```python
from build123d import *

# Parameters (mm, degrees)
F3_DEPTH = 15
F5_R     = 1
F6_DEPTH = 25


with BuildPart() as f1:
    # F0 (on Front) → F1 (revolve)
    with BuildSketch(Plane.XZ):
        with BuildLine():
            Line((2.6, 15), (2.6, 0))
            Line((2.6, 0), (21.5, 0))
            Line((21.5, 0), (21.5, 1))
            Line((21.5, 1), (20.5, 1))
            ThreePointArc((20.5, 1), (20.146447, 1.146447), (20, 1.5))
            Line((20, 1.5), (20, 13.5))
            ThreePointArc((20, 13.5), (20.146447, 13.853553), (20.5, 14))
            Line((20.5, 14), (21.5, 14))
            Line((21.5, 14), (21.5, 15))
            Line((21.5, 15), (2.6, 15))
        make_face()
    revolve(axis=Axis((0, 0, 3.375067), (0, 0, 1)))

    # F2 (on Top) → F3 (join, through all)
    with BuildSketch(Plane.XY):
        with BuildLine():
            Line((1.661325, -2), (-1.661325, -2))
            ThreePointArc((-1.661325, -2), (0, -2.6), (1.661325, -2))
        make_face()
    extrude(amount=F3_DEPTH)

    # F5 (on face) → F6 (cut)
    with BuildSketch(Plane(origin=(0, 6.5, 6.5), x_dir=(-1, 0, 0), z_dir=(0, 0.707107, 0.707107))):
        with Locations((0, 23.020815)):
            Circle(F5_R)
    extrude(amount=-F6_DEPTH, mode=Mode.SUBTRACT)


solid = f1.part
```
Could you check a few things on this model? Use its own coordinates, in mm. A direction names the side the tool comes from. Coordinates: 2 decimals unless noted, no trailing zeros. Write each loop counter-clockwise with the first axis right and the second up, starting at its lowest first coordinate (ties: lowest second). Pieces come first, ordered by that corner, then holes. Notation, with made-up numbers: (-14, 34) -> (31, 34) arc R28 cw to (31, 72) -> close; hole circle Ø11 at (32.25, 52.5). An arc over 180 degrees is marked (long way). Write item = value, one per line. Start each with the question number.
(1) I want a section at C-C (z = 7.5). Please give me the cut outline in (x, y), plus the area to 3 significant figures.
(2) Will these pins go through, and if not, where does the flat tip stop? pin 1 (1 mm diameter, centred on x = 7.5, z = 11.5, fed in from +Y) (3 decimals); pin 2 (2 mm diameter, centred on y = 8.5, z = 7, fed in from -X); pin 3 (8 mm diameter, centred on x = 2.5, z = 8.5, fed in from +Y).
(3) I need wall thicknesses on line 1 (Y direction, x = 0, z = 4); line 2 (X direction, y = 0, z = 11.25); line 3 (Z direction, x = -19, y = 8). Which ranges of each line are inside material? Lowest first, please. Write a range as [from, to].
(4) Which directions (+Z, -Z, +X, -X, +Y, -Y) give clear straight access to the entire face, cutting with the end or side of a thin tool? Please do faces 4 (the face through (4, 0, 15)), 5 (the face through (0, -2, 7)), 6 (the face through (0, -21, 1)).
(5) We'd pull the mould along X, two halves only. Please class faces 1 (the face through (-4.336, -19.524, 7.584)), 2 (the face through (-4, 0, 0)), 3 (the face through (0.1, 2.6, 7.4)): released by +X, released by -X, zero draft, split by the parting line, or undercut.
(6) I want a section at A-A (y = 0). Please give me the cut outline in (x, z), plus the area to 3 significant figures.
(7) I want a section at B-B (x = 0). Please give me the cut outline in (y, z).
Result set:
q1.outline = circle Ø40 at (0, 0); hole (-1.66, -2) -> (1.66, -2) arc R2.6 ccw (long way) to start
q1.area = 1,240 mm2
q2.pin_1 = 18.735
q2.pin_2 = -18.54
q2.pin_3 = 20
q3.line_1 = [-20, -2], [2.6, 20]
q3.line_2 = [-20, -2.6], [2.6, 20]
q3.line_3 = [0, 1], [14, 15]
q4.face_4 = +Z, +X, -X, +Y, -Y
q4.face_5 = +Z, -Z
q4.face_6 = none
q5.face_1 = split by the parting line
q5.face_2 = zero draft
q5.face_3 = undercut
q6.outline = (-21.5, 0) -> (-2.6, 0) -> (-2.6, 15) -> (-21.5, 15) -> (-21.5, 14) -> (-20.5, 14) arc R0.5 cw to (-20, 13.5) -> (-20, 1.5) arc R0.5 cw to (-20.5, 1) -> (-21.5, 1) -> close; (2.6, 0) -> (21.5, 0) -> (21.5, 1) -> (20.5, 1) arc R0.5 cw to (20, 1.5) -> (20, 13.5) arc R0.5 cw to (20.5, 14) -> (21.5, 14) -> (21.5, 15) -> (2.6, 15) -> close
q6.area = 528 mm2
q7.outline = (-21.5, 0) -> (-2, 0) -> (-2, 15) -> (-16.14, 15) -> (-20, 11.14) -> (-20, 1.5) arc R0.5 cw to (-20.5, 1) -> (-21.5, 1) -> close; (-21.5, 14) -> (-20.5, 14) arc R0.5 cw to (-20.13, 13.84) -> (-18.97, 15) -> (-21.5, 15) -> close; (2.6, 0) -> (21.5, 0) -> (21.5, 1) -> (20.5, 1) arc R0.5 cw to (20, 1.5) -> (20, 13.5) arc R0.5 cw to (20.5, 14) -> (21.5, 14) -> (21.5, 15) -> (2.6, 15) -> close
